Geometry: final body of the model. Coordinates: model frame, mm. A direction names the side the tool comes from. Round coordinates to 2 decimals unless told otherwise and drop trailing zeros. Write each loop counter-clockwise with the first axis right and the second up, starting at its lowest first coordinate (ties: lowest second). Pieces come first, ordered by that corner, then holes. Notation, with made-up numbers: M 78.25,25 L 103.25,25 A23 ccw 103.25,37 Z; hole C -39,56 d9. An arc over 180 degrees is marked long. Put each result on its own line as item: value. Start each with the question number.
```python
from build123d import *

# Parameters (mm, degrees)
SKETCH2_W           = 34
SKETCH2_H           = 34
SKETCH2_W_2         = 26.224899522
SKETCH2_H_2         = 26.224899522
BOSS_EXTRUDE1_DEPTH = 3.5
SKETCH4_W           = 19.088264776
SKETCH4_H           = 9.085831195
BOSS_EXTRUDE2_DEPTH = 4
FILLET1_R           = 8


with BuildPart() as part:
    # Sketch2 → Boss-Extrude1 (new body)
    # profile 1 of 2: a face of its own
    with BuildSketch(Plane.XY):
        Rectangle(SKETCH2_W, SKETCH2_H)
        Rectangle(SKETCH2_W_2, SKETCH2_H_2, mode=Mode.SUBTRACT)
    # profile 2 of 2: a face of its own
    with BuildSketch(Plane.XY):
        Polygon((4.976248984, 13.112449761), (-4.976248984, 13.112449761), (-4.976248984, 5.775025294), (-9.544132388, 5.775025294), (-9.544132388, -9.69135518), (9.544132388, -9.69135518), (9.544132388, 5.775025294), (4.976248984, 5.775025294), align=None)
    extrude(amount=BOSS_EXTRUDE1_DEPTH)

    # Sketch4 → Boss-Extrude2 (add)
    with BuildSketch(Plane.XY.offset(3.5)):
        with Locations((0, 1.232109697)):
            Rectangle(SKETCH4_W, SKETCH4_H)
    extrude(amount=BOSS_EXTRUDE2_DEPTH)

    # Fillet1
    fillet1_edges = [part.edges().sort_by_distance(p)[0] for p in [
        (-17, 17, 1.75),
        (17, 17, 1.75),
        (17, -17, 1.75),
        (-17, -17, 1.75),
    ]]
    fillet(fillet1_edges, radius=FILLET1_R)


solid = part.part
```
1) Ray query, probe 1 along Y at (x, z) = (-8.5, 1.5); probe 2 along X at (y, z) = (-6, 0.5); probe 3 along X at (y, z) = (12.5, 2.75). Return the intervals inside material, ascending.
2) Access query for faces 4 (the face through (14.594, 14.719, 1.774)), 5 (the face through (0, -6, 3.5)), 6 (the face through (9.544, 0, 3)). Directions: +Z, -Z, +X, -X, +Y, -Y. A direction counts if a zero-diameter tool reaches every point of the face in a straight line with its end or side. Return the directions, or none.
3) Section B-B, the plane y = 0. Output: boundary loops of the cut face in (x, z), and give its area (3 significant figures).
4) Draft query along Y for faces 1 (the face through (-4.976, 9, 2)), 2 (the face through (14.594, -14.719, 1.774)), 3 (the face through (17, 0, 2)). Return one class per face: +Y half, -Y half, draft (parallel to the pull), parting line (faces both ways), or undercut.
5) Section A-A, the plane x = 4.5. Output: boundary loops of the cut face in (y, z).
6) Section C-C, the plane z = 2.75. Output: boundary loops of the cut face in (x, y), and give its area (3 significant figures).
7) Section D-D, the plane y = -8. Output: boundary loops of the cut face in (x, z), and give its area (3 significant figures).
8) First-contact query: pin 1 (4 mm diameter, centred on x = 12, z = 5, fed in from -Y); pin 2 (3 mm diameter, centred on x = 4.5, z = 6, fed in from -Y); pin 3 (1 mm diameter, centred on x = -12.5, z = 3.5, fed in from +Y). Flat tips, straight axial feed; report the tip coordinate or a pass-through.
Solved:
1. probe 1: y = -17 to -13.11, -9.69 to 5.78, 13.11 to 17
1. probe 2: x = -17 to -13.11, -9.54 to 9.54, 13.11 to 17
1. probe 3: x = -16.19 to -13.11, -4.98 to 4.98, 13.11 to 16.19
2. face 4: +Z, -Z, +X, +Y
2. face 5: +Z, +X, -X, -Y
2. face 6: +Z, -Z
3. outline: M -17,0 L -13.11,0 L -13.11,3.5 L -17,3.5 Z; M -9.54,0 L 9.54,0 L 9.54,7.5 L -9.54,7.5 Z; M 13.11,0 L 17,0 L 17,3.5 L 13.11,3.5 Z
3. area: 170 mm2
4. face 1: undercut
4. face 2: -Y half
4. face 3: draft
5. outline: M -17,0 L -13.11,0 L -13.11,3.5 L -17,3.5 Z; M -9.69,0 L 17,0 L 17,3.5 L 5.78,3.5 L 5.78,7.5 L -3.31,7.5 L -3.31,3.5 L -9.69,3.5 Z
6. outline: M -17,-9 A8 ccw -9,-17 L 9,-17 A8 ccw 17,-9 L 17,9 A8 ccw 9,17 L -9,17 A8 ccw -17,9 Z; hole M -13.11,-13.11 L 13.11,-13.11 L 13.11,13.11 L 4.98,13.11 L 4.98,5.78 L 9.54,5.78 L 9.54,-9.69 L -9.54,-9.69 L -9.54,5.78 L -4.98,5.78 L -4.98,13.11 L -13.11,13.11 Z
6. area: 782 mm2
7. outline: M -17,0 L -13.11,0 L -13.11,3.5 L -17,3.5 Z; M -9.54,0 L 9.54,0 L 9.54,3.5 L -9.54,3.5 Z; M 13.11,0 L 17,0 L 17,3.5 L 13.11,3.5 Z
7. area: 94.0 mm2
8. pin 1: stops at y = -16.82
8. pin 2: stops at y = -3.31
8. pin 3: stops at y = 16.42
